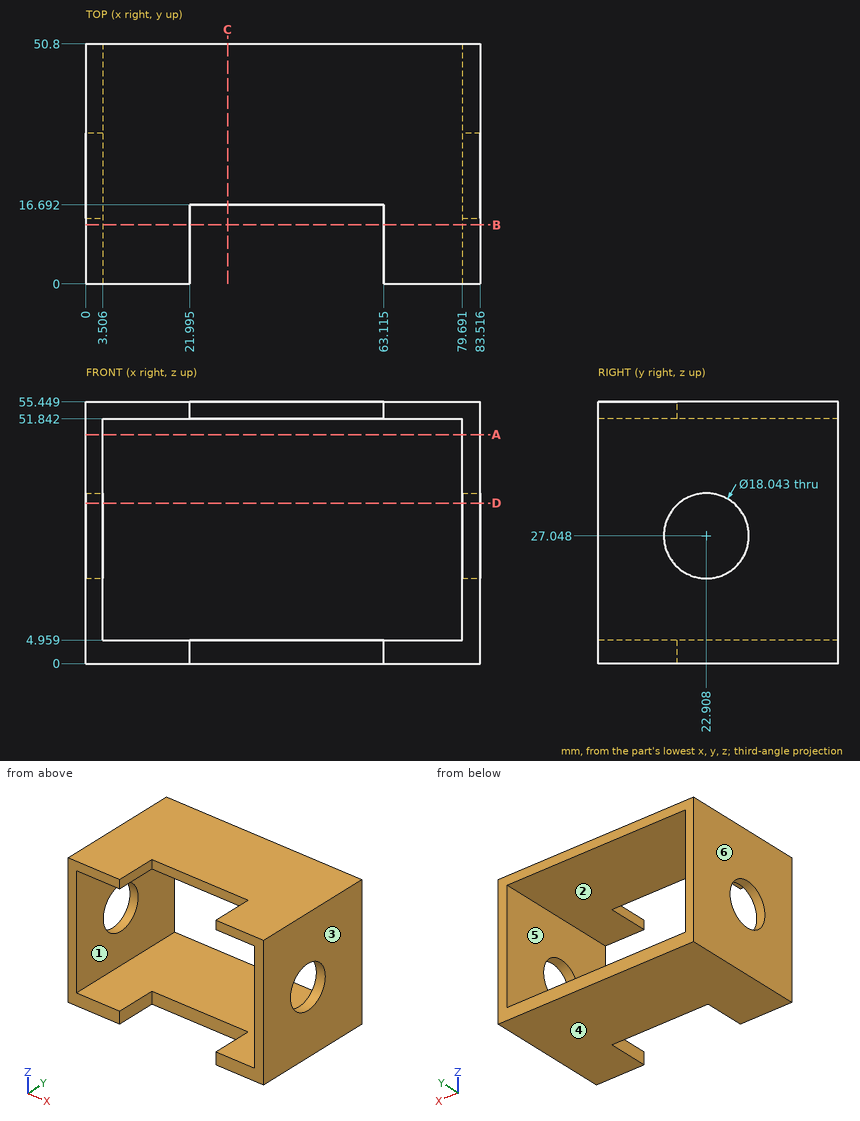
For this review, use the dimensioned drawing (mm, ordinates from the lowest corner) and the shaded views. A direction names the side the tool comes from. Coordinates: 2 decimals unless noted, no trailing zeros. Loops run counter-clockwise (first coordinate to the right, second up) from the corner with the lowest first, then second, coordinate; pieces in that order, holes last. Notation, with made-up numbers: (-18.5, 53) - (-13.5, 53) arc R13 cw to (-13.5, 68) - close; hole circle Ø5 at (33, 75). An arc over 180 degrees is marked (long way). Use CSV: the item, a comma, the result in double quotes. Start each with the question number.
1) The part is to be moulded in two halves that separate along X. For the marked faces 1, 2, 3 and 4, say which applies: +X half, -X half, draft (parallel to the pull), parting line (faces both ways), or undercut.
2) Consider section B-B on y = 12.5. Write out the cut boundary in (x, z) (1 decimal), then the cut area to 3 significant figures.
3) Consider section C-C on x = 30. Write out the cut boundary in (y, z), then the cut area to 3 significant figures.
4) For pin 1 Ø4 at (x, z) = (42, 2.5) entering from -Y, flat-tipped, find the tip position at first contact; note if it passes through.
5) Wall thickness on L1, parallel to Z at x = 25, y = 41.5; L2, parallel to X at y = 24, z = 12; L3, parallel to Y at x = 58, z = 3: over which ranges is each line inside the solid? List them lowest first. Write a range as from..to.
6) Consider section A-A on z = 48.5. Write out the cut boundary in (x, y).
7) Consider section D-D on z = 34. Write out the cut boundary in (x, y).
8) Tool access review of the marked faces 5 and 6: name each direction out of +Z, -Z, +X, -X, +Y, -Y from which nothing blocks a thin tool from reaching the whole face with its end or side.
Geometry says:
1,face 1,"undercut"
1,face 2,"undercut"
1,face 3,"+X half"
1,face 4,"draft"
2,outline,"(0, 0) - (22, 0) - (22, 5) - (3.5, 5) - (3.5, 51.8) - (22, 51.8) - (22, 55.4) - (0, 55.4) - close; (63.1, 0) - (83.5, 0) - (83.5, 55.4) - (63.1, 55.4) - (63.1, 51.8) - (79.7, 51.8) - (79.7, 5) - (63.1, 5) - close"
2,area,"707 mm^2"
3,outline,"(16.69, 0) - (50.8, 0) - (50.8, 4.96) - (16.69, 4.96) - close; (16.69, 51.84) - (50.8, 51.84) - (50.8, 55.45) - (16.69, 55.45) - close"
3,area,"292 mm^2"
4,pin 1,"y = 16.69"
5,L1,"0..4.96, 51.84..55.45"
5,L2,"0..3.51, 79.69..83.52"
5,L3,"16.69..50.8"
6,outline,"(0, 0) - (3.51, 0) - (3.51, 50.8) - (0, 50.8) - close; (79.69, 0) - (83.52, 0) - (83.52, 50.8) - (79.69, 50.8) - close"
7,outline,"(0, 0) - (3.51, 0) - (3.51, 17.16) - (0, 17.16) - close; (0, 28.66) - (3.51, 28.66) - (3.51, 50.8) - (0, 50.8) - close; (79.69, 0) - (83.52, 0) - (83.52, 17.16) - (79.69, 17.16) - close; (79.69, 28.66) - (83.52, 28.66) - (83.52, 50.8) - (79.69, 50.8) - close"
8,face 5,"+Y, -Y"
8,face 6,"+Z, -Z, -X, +Y, -Y"
